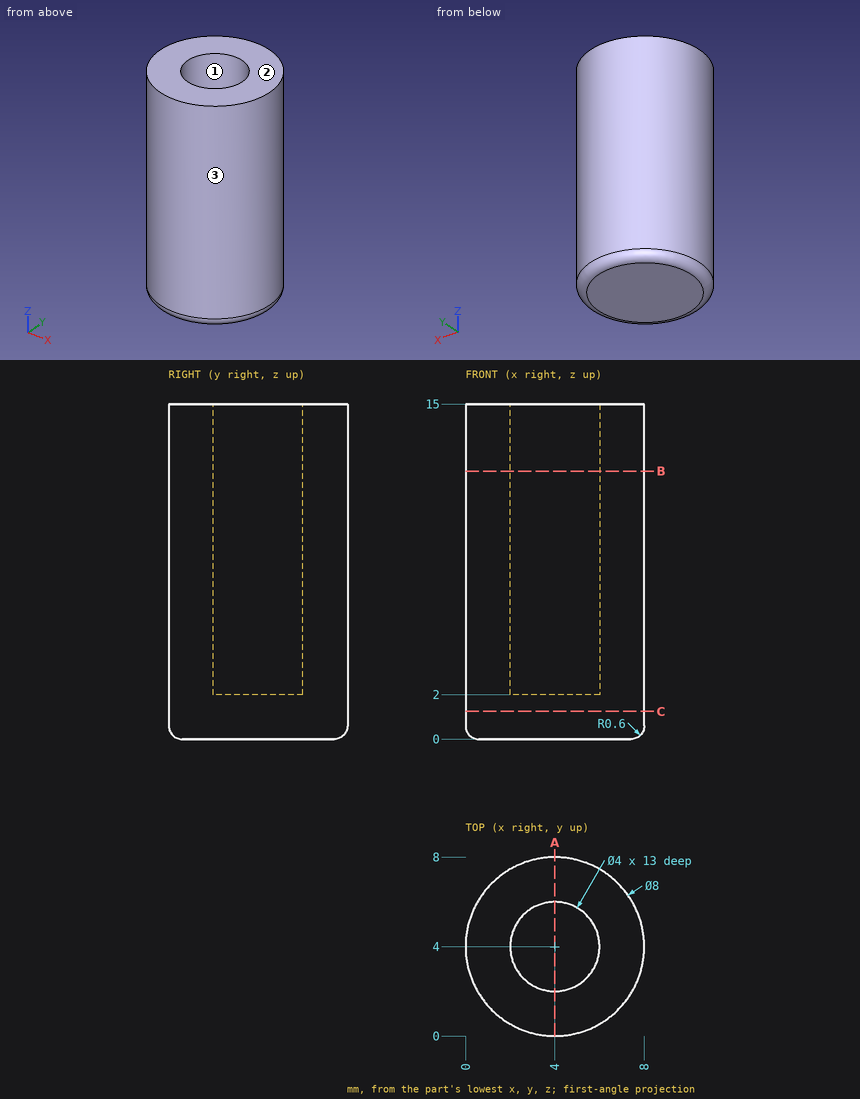
Drawing for the job (mm, zero at the part's lowest x, y, z). Round coordinates to 2 decimals unless told otherwise and drop trailing zeros. Write each loop counter-clockwise with the first axis right and the second up, starting at its lowest first coordinate (ties: lowest second). Pieces come first, ordered by that corner, then holes.
Item 1: Drill centre lines: L1, parallel to Y at x = 4, z = 5.5; L2, parallel to Z at x = 5, y = 4.75; L3, parallel to X at y = 4.75, z = 4.5. Where is each one in solid material? Low to high.
Filled in:
L1: y = 0 to 2, 6 to 8
L2: z = 0 to 2
L3: x = 0.07 to 2.15, 5.85 to 7.93
Item 2: Band-saw the part on B-B on z = 12. Write the cut outline in (x, y).
Filled in:
outline: circle Ø8 at (4, 4); hole circle Ø4 at (4, 4)
Item 3: Drop flat-ended pins along their axis: pin 1 Ø3 at (x, y) = (4, 4) entering from +Z; pin 2 Ø1 at (x, z) = (3, 3) entering from -Y; pin 3 Ø1.5 at (x, z) = (1, 8.5) entering from +Y. Give the stop position or say it passes through.
Filled in:
pin 1: stops at z = 2
pin 2: stops at y = 0.03
pin 3: stops at y = 7.31
Item 4: Band-saw the part on A-A on x = 4. Write the cut outline in (y, z), then the cut area to 3 significant figures.
Filled in:
outline: (0, 0.6) arc R0.6 ccw to (0.6, 0) - (7.4, 0) arc R0.6 ccw to (8, 0.6) - (8, 15) - (6, 15) - (6, 2) - (2, 2) - (2, 15) - (0, 15) - close
area: 67.8 mm2
Item 5: Band-saw the part on C-C on z = 1.25. Write the cut outline in (x, y), then the cut area to 3 significant figures.
Filled in:
outline: circle Ø8 at (4, 4)
area: 50.3 mm2
Item 6: Mould opens along Y. For the marked faces 1, 2 and 3 say: released by +Y, released by -Y, zero draft, split by the parting line, or undercut.
Filled in:
face 1: undercut
face 2: zero draft
face 3: split by the parting line
